Can you work these out from the model? Positions are in its coordinate system, mm. Face numbers are marked on the shaded views. A direction names the side the tool comes from. Round coordinates to 2 decimals unless told otherwise and drop trailing zeros. Loops run counter-clockwise (first coordinate to the right, second up) from the corner with the lowest first, then second, coordinate; pieces in that order, holes last. Notation, with made-up numbers: M 71,-37 L 98,-37 A6 cw 98,-27 Z; hole C 67.25,3.25 d8. An arc over 180 degrees is marked long. Return JSON: item names as keys, results as strings.
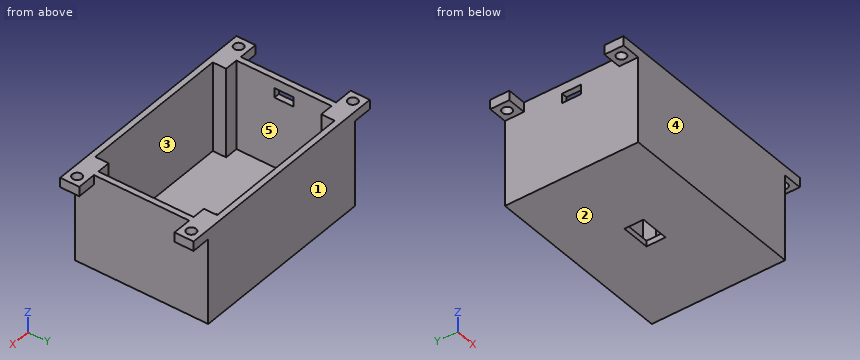
```python
from build123d import *

# Parameters (mm, degrees)
ESQUISSE1_W             = 100
ESQUISSE1_H             = 70
BOSS_EXTRU_1_DEPTH      = 50
ESQUISSE2_W             = 94
ESQUISSE2_H             = 64
ENL_V_MAT_EXTRU_1_DEPTH = 47
ESQUISSE4_W             = 15
ESQUISSE4_H             = 10
ENL_V_MAT_EXTRU_3_DEPTH = 47
ESQUISSE5_W             = 20
ESQUISSE5_H             = 10
BOSS_EXTRU_2_DEPTH      = 50
ESQUISSE6_W             = 10
ESQUISSE6_H             = 10
ENL_V_MAT_EXTRU_4_DEPTH = 45
ESQUISSE7_R             = 2.5
ENL_V_MAT_EXTRU_5_DEPTH = 45
ESQUISSE3_W             = 5
ESQUISSE3_H             = 10
ENL_V_MAT_EXTRU_6_DEPTH = 45


with BuildPart() as part:
    # Esquisse1 → Boss.-Extru.1 (new body)
    with BuildSketch(Plane.XY):
        with Locations((-50, 35)):
            Rectangle(ESQUISSE1_W, ESQUISSE1_H)
    extrude(amount=BOSS_EXTRU_1_DEPTH)

    # Esquisse2 → Enlèv. mat.-Extru.1 (cut)
    with BuildSketch(Plane.XY.offset(50)):
        with Locations((-50, 35)):
            Rectangle(ESQUISSE2_W, ESQUISSE2_H)
    extrude(amount=-ENL_V_MAT_EXTRU_1_DEPTH, mode=Mode.SUBTRACT)

    # Esquisse4 → Enlèv. mat.-Extru.3 (cut)
    with BuildSketch(Plane(origin=(0, 0, 0), x_dir=(-1, 0, 0), z_dir=(0, 0, -1))):
        with Locations((50, 35)):
            Rectangle(ESQUISSE4_W, ESQUISSE4_H)
    extrude(amount=-ENL_V_MAT_EXTRU_3_DEPTH, mode=Mode.SUBTRACT)

    # Esquisse5 → Boss.-Extru.2 (add)
    with BuildSketch(Plane(origin=(0, 0, 0), x_dir=(-1, 0, 0), z_dir=(0, 0, -1))):
        with Locations((0, 5)):
            Rectangle(ESQUISSE5_W, ESQUISSE5_H)
        with Locations((0, 65)):
            Rectangle(ESQUISSE5_W, ESQUISSE5_H)
        with Locations((100, 5)):
            Rectangle(ESQUISSE5_W, ESQUISSE5_H)
        with Locations((100, 65)):
            Rectangle(ESQUISSE5_W, ESQUISSE5_H)
    extrude(amount=-BOSS_EXTRU_2_DEPTH)

    # Esquisse6 → Enlèv. mat.-Extru.4 (cut)
    with BuildSketch(Plane(origin=(0, 0, 0), x_dir=(-1, 0, 0), z_dir=(0, 0, -1))):
        with Locations((-5, 65)):
            Rectangle(ESQUISSE6_W, ESQUISSE6_H)
        with Locations((-5, 5)):
            Rectangle(ESQUISSE6_W, ESQUISSE6_H)
        with Locations((105, 65)):
            Rectangle(ESQUISSE6_W, ESQUISSE6_H)
        with Locations((105, 5)):
            Rectangle(ESQUISSE6_W, ESQUISSE6_H)
    extrude(amount=-ENL_V_MAT_EXTRU_4_DEPTH, mode=Mode.SUBTRACT)

    # Esquisse7 → Enlèv. mat.-Extru.5 (cut)
    with BuildSketch(Plane(origin=(0, 0, 45), x_dir=(-1, 0, 0), z_dir=(0, 0, -1))):
        with Locations((-5, 65)):
            Circle(ESQUISSE7_R)
        with Locations((-5, 5)):
            Circle(ESQUISSE7_R)
        with Locations((105, 5)):
            Circle(ESQUISSE7_R)
        with Locations((105, 65)):
            Circle(ESQUISSE7_R)
    extrude(amount=-ENL_V_MAT_EXTRU_5_DEPTH, mode=Mode.SUBTRACT)

    # Esquisse3 → Enlèv. mat.-Extru.6 (cut)
    with BuildSketch(Plane.ZY.offset(100)):
        with Locations((42.5, 35)):
            Rectangle(ESQUISSE3_W, ESQUISSE3_H)
    extrude(amount=-ENL_V_MAT_EXTRU_6_DEPTH, mode=Mode.SUBTRACT)


solid = part.part
```
Q1. Suppose I cut it at A-A, the plane x = 5. Please give me the cut outline in (y, z), plus the area to 3 significant figures.
Results:
{"outline": "M 0,45 L 2.5,45 L 2.5,50 L 0,50 Z; M 7.5,45 L 10,45 L 10,50 L 7.5,50 Z; M 60,45 L 62.5,45 L 62.5,50 L 60,50 Z; M 67.5,45 L 70,45 L 70,50 L 67.5,50 Z", "area": "50.0 mm2"}
Q2. Suppose I cut it at D-D, the plane x = -65. Please give me the cut outline in (y, z).
Results:
{"outline": "M 0,0 L 70,0 L 70,50 L 67,50 L 67,3 L 3,3 L 3,50 L 0,50 Z"}
Q3. I'm going to push flat-ended pins straight in: pin 1 Ø3 at (y, z) = (27, 19.5) entering from -X; pin 2 Ø25 at (y, z) = (37, 19) entering from +X; pin 3 Ø3 at (x, y) = (-34, 42.5) entering from +Z. Where does each tip first touch, or does it pass through?
Results:
{"pin 1": "stops at x = -100", "pin 2": "stops at x = 0", "pin 3": "stops at z = 3"}
Q4. Suppose I cut it at B-B, the plane z = 9. Please give me the cut outline in (x, y), plus the area to 3 significant figures.
Results:
{"outline": "M -100,0 L 0,0 L 0,70 L -100,70 Z; hole M -97,10 L -90,10 L -90,3 L -10,3 L -10,10 L -3,10 L -3,60 L -10,60 L -10,67 L -90,67 L -90,60 L -97,60 Z", "area": "1,180 mm2"}
Q5. Suppose I cut it at C-C, the plane y = 5. Please give me the cut outline in (x, z), plus the area to 3 significant figures.
Results:
{"outline": "M -110,45 L -107.5,45 L -107.5,50 L -110,50 Z; M -102.5,45 L -100,45 L -100,0 L 0,0 L 0,45 L 2.5,45 L 2.5,50 L -10,50 L -10,3 L -90,3 L -90,50 L -102.5,50 Z; M 7.5,45 L 10,45 L 10,50 L 7.5,50 Z", "area": "1,290 mm2"}
Q6. If I drill on line 1 along Y through (x, z) = (-105, 48.05); line 2 along Y through (x, z) = (-44, 39); line 3 along X through (y, z) = (47.5, 16.5), over which ranges is the centre line in solid material (lowest first)?
Results:
{"line 1": "y = 0 to 2.5, 7.5 to 10, 60 to 62.5, 67.5 to 70", "line 2": "y = 0 to 3, 67 to 70", "line 3": "x = -100 to -97, -3 to 0"}
Q7. Thinking about a two-plate mould opening in Y: for the marked faces 1, 2 and 3, which applies, pulls with the +Y half, pulls with the -Y half, needs draft (parallel to the pull), parting line crosses it, or undercut?
Results:
{"face 1": "pulls with the +Y half", "face 2": "needs draft", "face 3": "undercut"}
Q8. On a 3-axis mill with a long thin cutter (end or side, diameter ignored), from which of +Z, -Z, +X, -X, +Y, -Y can I reach the whole of each face in a straight line? I mean the marked faces 4 and 5. Say none if no direction works.
Results:
{"face 4": "+Z, -Z, +X, -X, -Y", "face 5": "+Z"}
